Source: CAD feature listing. Evaluate the final solid. Frame: model axes, mm. A direction names the side the tool comes from. Coordinates: 2 decimals unless noted, no trailing zeros. Write each loop counter-clockwise with the first axis right and the second up, starting at its lowest first coordinate (ties: lowest second). Pieces come first, ordered by that corner, then holes. Notation, with made-up numbers: M -38,22.5 L 0,22.5 A5 cw 0,28.5 Z; hole C 32,28 d4. An arc over 180 degrees is marked long. One line per item, written item: value. Start each with the question number.
Item 1: Mould query, pull axis X, two halves, no side actions, for faces 1 (the flat face through (16.7, 0, -15)), 2 (the cylindrical face through (18.3, 0.6, -17.1)), 3 (the flat face through (18, 0, -20.65)), 4 (the flat face through (4.5, -1, 0)). Classes: released by +X, released by -X, zero draft, split by the parting line, or undercut.
Item 2: Cut plane C-C, the plane z = -12. Output: boundary loops of the cut face in (x, y), then the cut area to 3 significant figures.
Item 3: Pin query (flat end, axial travel): P1, Ø1.2, axis at y = -0.5, z = 0.5, coming from the -X side; P2, Ø1.5, axis at x = 15.5, y = -2.5, coming from the +Z side; P3, Ø1.2, axis at x = 19.05, y = 0.6, coming from the -Z side. Return the tip coordinate at first contact, or that it passes through.
Item 4: Ray query, L1, parallel to X at y = 0.6, z = -18.5; L2, parallel to Y at x = -2.25, z = 0; L3, parallel to X at y = 2.75, z = -10.5. Return the intervals inside material, ascending. Write a range as from..to.
Item 5: Cut plane D-D, the plane x = 0. Output: boundary loops of the cut face in (y, z), then the cut area to 3 significant figures.
Item 6: Cut plane A-A, the plane y = -0.6. Output: boundary loops of the cut face in (x, z) (3 decimals).
Item 7: Set-up query: faces 5 (the cylindrical face through (-3.308, -2.552, 0.434)), 6 (the flat face through (5, 0, -5.5)), 7 (the cylindrical face through (-9.5, 0.6, -17.1)). Return all of +Z, -Z, +X, -X, +Y, -Y with unobstructed straight access to the full face (end or side cutting, diameter ignored); none if empty.
Item 8: Cut plane B-B, the plane z = -19. Output: boundary loops of the cut face in (x, y).
```python
from build123d import *

# Parameters (mm, degrees)
BOSS_EXTRUDE1_DEPTH            = 4
FILLET1_R                      = 3.175
CUT_EXTRUDE1_DEPTH             = 30.864067037
CUT_EXTRUDE1_DEPTH_BACK        = 30.864067037
SKETCH2_R                      = 2
CUT_EXTRUDE2_DEPTH             = 4.5
CUT_EXTRUDE2_DEPTH_BACK        = 30.864067037
SKETCH3_R                      = 2
F_1_5_1_5_DIAMETER_HOLE1_D     = 1.5
F_1_5_1_5_DIAMETER_HOLE1_DEPTH = 7
F_1_5_1_5_DIAMETER_HOLE1_TIP   = 0.450645464
CBORE_FOR_M3_SHCS1_D           = 3.2
CBORE_FOR_M3_SHCS1_CBORE_D     = 6.5
CBORE_FOR_M3_SHCS1_CBORE_DEPTH = 3


with BuildPart() as part:
    # Sketch1 → Boss-Extrude1 (new, symmetric)
    with BuildSketch(Plane(origin=(0, 0, 0), x_dir=(1, 0, 0), z_dir=(0, 1, 0))):
        Polygon((12, 0.5), (12, -6), (-10.9, -6), (-10.9, 20.65), (-6.4, 20.65), (-6.4, 5.5), (16.7, 5.5), (16.7, 20.65), (21.2, 20.65), (21.2, 0.5), align=None)
    extrude(amount=BOSS_EXTRUDE1_DEPTH, both=True)

    # Fillet1
    fillet1_edges = [part.edges().sort_by_distance(p)[0] for p in [
        (12, 0, -0.5),
        (-6.4, 0, -5.5),
        (16.7, 0, -5.5),
    ]]
    fillet(fillet1_edges, radius=FILLET1_R)

    # Sketch2 → Cut-Extrude1 (cut, two sides: drawn at the far end of the back side and taken through both)
    with BuildSketch(Plane.XY.offset(-CUT_EXTRUDE1_DEPTH_BACK)):
        with Locations((0, 0.6)):
            Circle(SKETCH2_R)
    extrude(amount=CUT_EXTRUDE1_DEPTH + CUT_EXTRUDE1_DEPTH_BACK, mode=Mode.SUBTRACT)

    # Sketch3 → Cut-Extrude2 (cut, two sides: drawn at the far end of the back side and taken through both)
    with BuildSketch(Plane(origin=(0, 0, 0), x_dir=(0, 0, -1), z_dir=(1, 0, 0)).offset(-CUT_EXTRUDE2_DEPTH_BACK)):
        with Locations((0, -0.6)):
            Circle(SKETCH3_R)
    extrude(amount=CUT_EXTRUDE2_DEPTH + CUT_EXTRUDE2_DEPTH_BACK, mode=Mode.SUBTRACT)

    # Ø1.5 (1.5) Diameter Hole1
    with Locations(Plane(origin=(0, 0, -20.65), x_dir=(-1, 0, 0), z_dir=(0, 0, -1))):
        with Locations((-19.05, 0.6), (8.75, 0.6)):
            Hole(F_1_5_1_5_DIAMETER_HOLE1_D / 2, depth=F_1_5_1_5_DIAMETER_HOLE1_DEPTH)
            with Locations((0, 0, -(F_1_5_1_5_DIAMETER_HOLE1_DEPTH + F_1_5_1_5_DIAMETER_HOLE1_TIP / 2))):  # 118° drill point
                Cone(0, F_1_5_1_5_DIAMETER_HOLE1_D / 2, F_1_5_1_5_DIAMETER_HOLE1_TIP, mode=Mode.SUBTRACT)

    # CBORE for M3 SHCS1 (through all)
    with Locations(Plane(origin=(0, 4, 0), x_dir=(1, 0, 0), z_dir=(0, 1, 0))):
        with Locations((8, 0)):
            CounterBoreHole(CBORE_FOR_M3_SHCS1_D / 2, CBORE_FOR_M3_SHCS1_CBORE_D / 2, CBORE_FOR_M3_SHCS1_CBORE_DEPTH)


solid = part.part
```
From the geometry:
1. face 1: undercut
1. face 2: undercut
1. face 3: zero draft
1. face 4: released by -X
2. outline: M -10.9,-4 L -6.4,-4 L -6.4,4 L -10.9,4 Z; M 16.7,-4 L 21.2,-4 L 21.2,4 L 16.7,4 Z
2. area: 72.0 mm²
3. P1: stops at x = 4.5
3. P2: stops at z = -0.47
3. P3: stops at z = -13.56
4. L1: x = -10.9..-9.5, -8..-6.4, 16.7..18.3, 19.8..21.2
4. L2: y = -4..-2.6, 1.4..4
4. L3: x = -10.9..-6.4, 16.7..21.2
5. outline: M -4,-5.5 L -1.4,-5.5 L -1.4,-1.83 A2 cw -1.4,1.83 L -1.4,6 L -4,6 Z; M 2.6,-5.5 L 4,-5.5 L 4,6 L 2.6,6 Z
5. area: 42.8 mm²
6. outline: M -10.9,-20.65 L -6.4,-20.65 L -6.4,-8.675 A3.175 cw -3.225,-5.5 L -1.6,-5.5 L -1.6,-2 L -10.9,-2 Z; M -10.9,2 L -1.6,2 L -1.6,6 L -10.9,6 Z; M 1.6,-5.5 L 13.525,-5.5 A3.175 cw 16.7,-8.675 L 16.7,-20.65 L 21.2,-20.65 L 21.2,-0.5 L 15.175,-0.5 A3.175 cw 12,2.675 L 12,6 L 1.6,6 L 1.6,2 L 4.5,2 L 4.5,-2 L 1.6,-2 Z; hole C 8,0 d3.2
7. face 5: -X
7. face 6: -Z, +Y, -Y
7. face 7: -Z
8. outline: M -10.9,-4 L -6.4,-4 L -6.4,4 L -10.9,4 Z; M 16.7,-4 L 21.2,-4 L 21.2,4 L 16.7,4 Z; hole C -8.75,0.6 d1.5; hole C 19.05,0.6 d1.5
